Study the drawing (mm; zero at the part's minimum x, y, z) and answer. Give positions to 0.01 mm unless a question says otherwise; leave off trailing zeros. Order: outer loops, then holes, each group sorted by start corner. A loop starts at its lowest first (then second) coordinate and runs counter-clockwise, first axis right, second up. Notation, with made-up numbers: (3, 13) - (50, 13) arc R25 cw to (50, 35) - close; hole circle Ø5 at (73, 15). An arc over 180 degrees is marked (long way). Write each question's results on one line, items separated by ' | '. Start each with the question number.
1. Section C-C (x = 6.5) is taken. Give the vertices of the cut face in (y, z), and give its area (3 significant figures).
2. Section A-A (y = 6.5) is taken. Give the vertices of the cut face in (x, z), and give its area (3 significant figures).
3. Section B-B (z = 19.5) is taken. Give the vertices of the cut face in (x, y).
4. Find the intervals of material crossed by L1, parallel to Y at x = 7.5, z = 23; L2, parallel to Y at x = 3.25, z = 10.25, in increasing order.
5. Determine the mould class of the marked faces 1, 2, 3 and 4 for opening direction Z: released by +Z, released by -Z, zero draft, split by the parting line, or undercut.
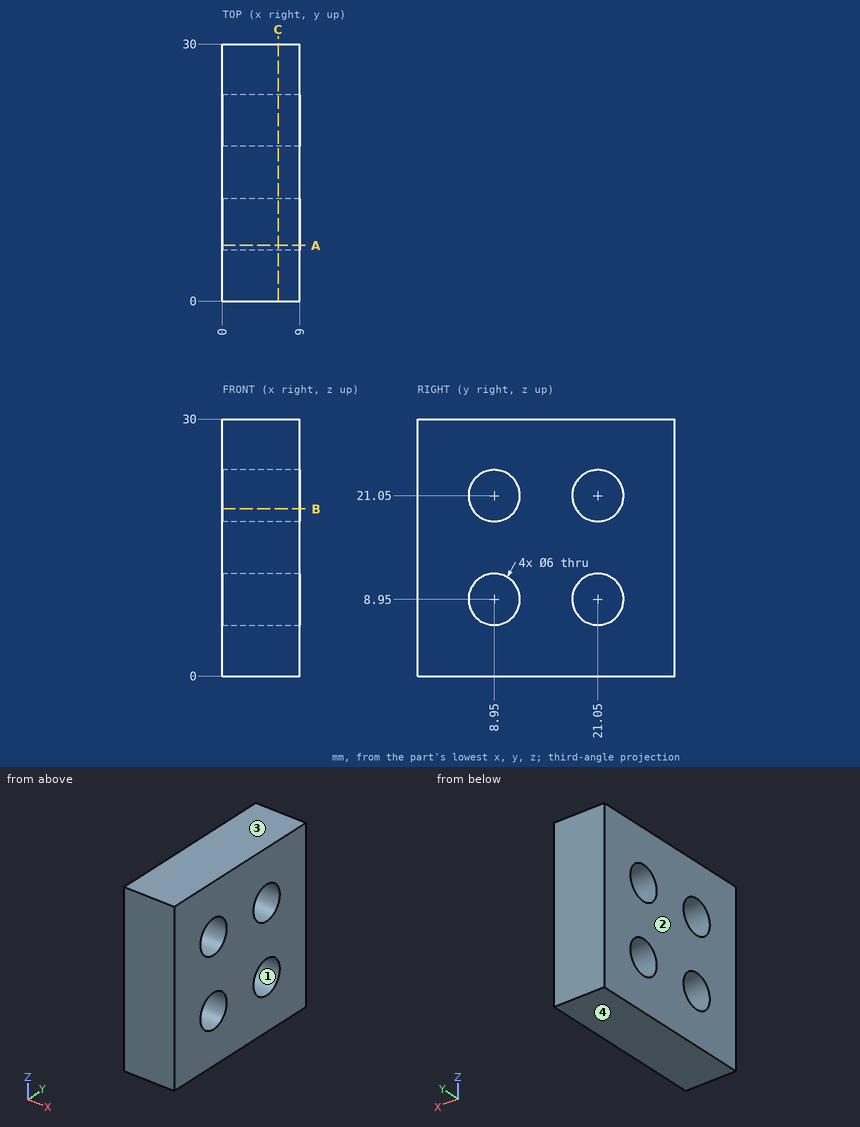
Reported:
1) outline: (0, 0) - (30, 0) - (30, 30) - (0, 30) - close; hole circle Ø6 at (8.95, 8.95); hole circle Ø6 at (8.95, 21.05); hole circle Ø6 at (21.05, 8.95); hole circle Ø6 at (21.05, 21.05) | area: 787 mm²
2) outline: (0, 0) - (9, 0) - (9, 7.22) - (0, 7.22) - close; (0, 10.68) - (9, 10.68) - (9, 19.32) - (0, 19.32) - close; (0, 22.78) - (9, 22.78) - (9, 30) - (0, 30) - close | area: 208 mm²
3) outline: (0, 0) - (9, 0) - (9, 6.38) - (0, 6.38) - close; (0, 11.52) - (9, 11.52) - (9, 18.48) - (0, 18.48) - close; (0, 23.62) - (9, 23.62) - (9, 30) - (0, 30) - close
4) L1: 0 to 6.67, 11.23 to 18.77, 23.33 to 30 | L2: 0 to 6.25, 11.65 to 18.35, 23.75 to 30
5) face 1: undercut | face 2: zero draft | face 3: released by +Z | face 4: released by -Z
